from build123d import *

# Parameters (mm, degrees)
SKETCH_1_W          = 54
SKETCH_1_H          = 4
EXTRUDE_2_DEPTH     = 3.5
SKETCH_2_W          = 60
SKETCH_2_H          = 11
EXTRUDE_3_DEPTH     = 5
SKETCH_3_W          = 60
SKETCH_3_H          = 3
CUT_EXTRUDE_1_DEPTH = 10
SKETCH_4_W          = 60
SKETCH_4_H          = 8
EXTRUDE_4_DEPTH     = 15
SKETCH_5_R          = 2.25
CUT_EXTRUDE_2_DEPTH = 64.749509802


with BuildPart() as part:
    # 스케치1 → 보스-돌출2 (new body)
    with BuildSketch(Plane.XY):
        with Locations((30, 2)):
            Rectangle(SKETCH_1_W, SKETCH_1_H)
    extrude(amount=EXTRUDE_2_DEPTH)

    # 스케치2 → 보스-돌출3 (add)
    with BuildSketch(Plane(origin=(0, 0, 0), x_dir=(-1, 0, 0), z_dir=(0, 0, -1))):
        with Locations((-30, 2.5)):
            Rectangle(SKETCH_2_W, SKETCH_2_H)
    extrude(amount=EXTRUDE_3_DEPTH)

    # 스케치3 → 컷-돌출1 (cut)
    with BuildSketch(Plane.XY):
        with Locations((30, -1.5)):
            Rectangle(SKETCH_3_W, SKETCH_3_H)
    extrude(amount=-CUT_EXTRUDE_1_DEPTH, mode=Mode.SUBTRACT)

    # 스케치4 → 보스-돌출4 (add)
    with BuildSketch(Plane(origin=(0, 0, -5), x_dir=(-1, 0, 0), z_dir=(0, 0, -1))):
        with Locations((-30, 4)):
            Rectangle(SKETCH_4_W, SKETCH_4_H)
    extrude(amount=EXTRUDE_4_DEPTH)

    # 스케치5 → 컷-돌출2 (cut, through all)
    with BuildSketch(Plane(origin=(0, 8, 0), x_dir=(1, 0, 0), z_dir=(0, 1, 0))):
        with Locations(Location((30, 12.5, 0), (0, 0, 270))):
            Circle(SKETCH_5_R)
    extrude(amount=-CUT_EXTRUDE_2_DEPTH, mode=Mode.SUBTRACT)


solid = part.part
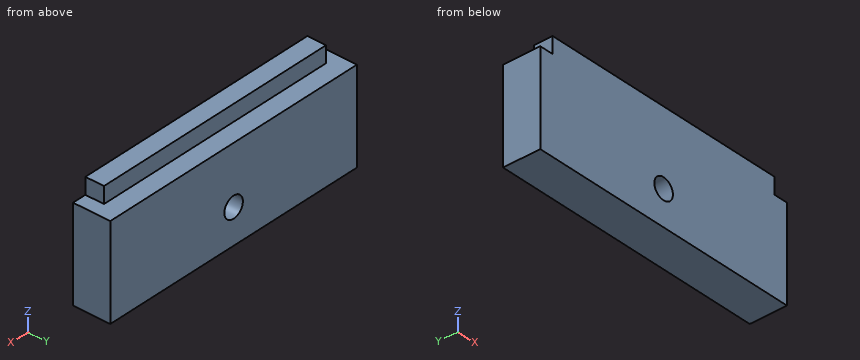
Verification items for the finished model (mm, model axes). Round coordinates to 2 decimals unless told otherwise and drop trailing zeros. Order: outer loops, then holes, each group sorted by start corner. A loop starts at its lowest first (then second) coordinate and runs counter-clockwise, first axis right, second up.
1. Section check A-A on x = 30. Record the cut outline in (y, z).
Final values:
outline: (0, -20) - (8, -20) - (8, -14.75) - (0, -14.75) - close; (0, -10.25) - (8, -10.25) - (8, 0) - (4, 0) - (4, 3.5) - (0, 3.5) - close
2. Section check C-C on y = 1.75. Record the cut outline in (x, z).
Final values:
outline: (0, -20) - (60, -20) - (60, 0) - (57, 0) - (57, 3.5) - (3, 3.5) - (3, 0) - (0, 0) - close; hole circle Ø4.5 at (30, -12.5)
3. Go/stop test with flat-tipped pins: P1, Ø3, axis at y = 1.5, z = 2, coming from the +X side; P2, Ø8, axis at x = 33.5, z = 0.5, coming from the -Y side; P3, Ø4, axis at y = 2, z = 2.5, coming from the -X side. Record where each tip stops, or that it passes through.
Final values:
P1: stops at x = 57
P2: stops at y = 0
P3: stops at x = 3
4. Section check D-D on y = 7. Record the cut outline in (x, z), then the cut area to 3 significant figures.
Final values:
outline: (0, -20) - (60, -20) - (60, 0) - (0, 0) - close; hole circle Ø4.5 at (30, -12.5)
area: 1,180 mm2
5. Section check B-B on z = -12.5. Record the cut outline in (x, y), then the cut area to 3 significant figures.
Final values:
outline: (0, 0) - (27.75, 0) - (27.75, 8) - (0, 8) - close; (32.25, 0) - (60, 0) - (60, 8) - (32.25, 8) - close
area: 444 mm2
6. Thickness scan on L1, parallel to X at y = 6, z = -12.5; L2, parallel to Z at x = 52.5, y = 5.5; L3, parallel to X at y = 0.5, z = -10.75. Record the ranges inside material, lowest first.
Final values:
L1: x = 0 to 27.75, 32.25 to 60
L2: z = -20 to 0
L3: x = 0 to 28.59, 31.41 to 60
